Input: part model. Units: mm. Frame: model coordinates. A direction names the side the tool comes from. Round coordinates to 2 decimals unless told otherwise and drop trailing zeros. Loops run counter-clockwise (first coordinate to the right, second up) from the corner with the lowest first, then second, coordinate; pieces in that order, holes last. Notation, with made-up numbers: M 76.25,54 L 110.25,54 A15 ccw 110.25,67 Z; hole C 14.5,-29.5 d5. An arc over 180 degrees is marked long. Return JSON: item names as keys, results as strings. Group by question number.
1) Section A-A (y = 0). Output: boundary loops of the cut face in (x, z).
2) Mould query, pull axis Y, two halves, no side actions, for faces 5 (the face through (-1.73, -7.81, 0.99)), 6 (the face through (3.98, -5.47, 0.99)), 7 (the face through (0, -42, 12)), 8 (the face through (-4.52, 3.03, 0.99)). Classes: +Y half, -Y half, draft (parallel to the pull), parting line (faces both ways), or undercut.
3) Material intervals for line 1 (Y direction, x = -4.25, z = 0.5); line 2 (Z direction, x = -4.5, y = -40); line 3 (X direction, y = -6, z = 9.75), sorted ascending. Write a range as from..to.
4) Access query for faces 1 (the face through (0, 7.5, 3)), 2 (the face through (-2, -2, 6)), 3 (the face through (0, -7.5, 3)), 4 (the face through (2, -2, 6)). Directions: +Z, -Z, +X, -X, +Y, -Y. A direction counts if a zero-diameter tool reaches every point of the face in a straight line with its end or side. Return the directions, or none.
5) Contact query for flat-ended pins moving along their axis: P1, Ø8, axis at x = 3.5, y = -28, coming from the -Z side; P2, Ø6.5, axis at y = -37.5, z = 7, coming from the -X side; P3, Ø1, axis at x = 6, z = 3, coming from the -Y side; P4, Ø1.5, axis at y = -29.5, z = 4, coming from the +X side. Output: stop coordinate, or through.
6) Section B-B (x = -4.25). Count the separate pieces of the cut face and the enclosed holes in it, plus the area to 3 significant figures.
from build123d import *

# Parameters (mm, degrees)
SKETCH_R     = 8
SKETCH_R_2   = 1.25
PAD_DEPTH    = 2
SKETCH001_W  = 4
SKETCH001_H  = 15
PAD001_DEPTH = 10
SKETCH002_W  = 4
SKETCH002_H  = 8
PAD002_DEPTH = 30
POCKET_DEPTH = 5
PAD003_DEPTH = 8


with BuildPart() as part:
    # Sketch → Pad (new body)
    with BuildSketch(Plane.XY):
        Circle(SKETCH_R)
        with Locations((-4.25, 4.25)):
            Circle(SKETCH_R_2, mode=Mode.SUBTRACT)
        with Locations((4.25, 4.25)):
            Circle(SKETCH_R_2, mode=Mode.SUBTRACT)
        with Locations((4.25, -4.25)):
            Circle(SKETCH_R_2, mode=Mode.SUBTRACT)
        with Locations((-4.25, -4.25)):
            Circle(SKETCH_R_2, mode=Mode.SUBTRACT)
    extrude(amount=PAD_DEPTH)

    # Sketch001 (on Face7 of Pad) → Pad001 (join)
    with BuildSketch(Plane.XY.offset(2)):
        Rectangle(SKETCH001_W, SKETCH001_H)
    extrude(amount=PAD001_DEPTH)

    # Sketch002 (on Face9 of Pad001) → Pad002 (join)
    with BuildSketch(Plane.XZ.offset(7.5)):
        with Locations((0, 8)):
            Rectangle(SKETCH002_W, SKETCH002_H)
    extrude(amount=PAD002_DEPTH)

    # Sketch003 (on Face10 of Pad002) → Pocket (cut)
    with BuildSketch(Plane.YZ.offset(2)):
        Polygon((-7.5, 12), (7.5, 4), (17.5, 4), (17.5, 22), (-7.5, 22), align=None)
    extrude(amount=-POCKET_DEPTH, mode=Mode.SUBTRACT)

    # Sketch004 (on Face16 of Pocket) → Pad003 (join)
    with BuildSketch(Plane.XY.offset(12)):
        with BuildLine():
            Line((-2, -7.5), (2, -7.5))
            Line((2, -7.5), (6, -17.5))
            Line((6, -17.5), (6, -37.5))
            add(Edge.make_bspline(
                [(6, -37.5), (6, -77.5), (-6, -77.5)],
                knots=[0, 0, 0, 1, 1, 1], degree=2))
            Line((-6, -77.5), (-6, -17.5))
            Line((-6, -17.5), (-2, -7.5))
        make_face()
    extrude(amount=-PAD003_DEPTH)


solid = part.part
Returned:
{
 "1": {"outline": "M -8,0 L 8,0 L 8,2 L 2,2 L 2,8 L -2,8 L -2,2 L -8,2 Z"},
 "2": {"face 5": "parting line", "face 6": "undercut", "face 7": "draft", "face 8": "undercut"},
 "3": {"line 1": "y = -6.78..-5.5, -3..3, 5.5..6.78", "line 2": "z = 4..12", "line 3": "x = -2..2"},
 "4": {"face 1": "+Z, +X, -X, +Y", "face 2": "+Z, -X, +Y", "face 3": "+X, -X, -Y", "face 4": "+Z, +X, +Y"},
 "5": {"P1": "stops at z = 4", "P2": "stops at x = -6", "P3": "passes through", "P4": "stops at x = 6"},
 "6": {"separate pieces": "4", "enclosed holes": "0", "area": "530 mm^2"}
}
